Part model, mm, in its own coordinate system. A direction names the side the tool comes from. Round coordinates to 2 decimals unless told otherwise and drop trailing zeros. Write each loop counter-clockwise with the first axis right and the second up, starting at its lowest first coordinate (ties: lowest second). Pieces come first, ordered by that corner, then holes.
from build123d import *

# Parameters (mm, degrees)
F1_DEPTH = 5
F2_W     = 30
F2_H     = 15
F3_DEPTH = 3
F4_R     = 5.490381
F4_R_2   = 3
F5_DEPTH = 8


with BuildPart() as f1:
    # F0 (on Top) → F1 (new body)
    with BuildSketch(Plane.XY):
        Polygon((0, 25.980762), (-15, 0), (15, 0), align=None)
    extrude(amount=F1_DEPTH)

    # F2 (on face) → F3 (join)
    with BuildSketch(Plane.XZ):
        with Locations((0, 7.5)):
            Rectangle(F2_W, F2_H)
    extrude(amount=F3_DEPTH)

    # F4 (on face) → F5 (join)
    with BuildSketch(Plane.XY.offset(5)):
        with Locations((0, 15)):
            Circle(F4_R)
        with Locations((0, 15)):
            Circle(F4_R_2, mode=Mode.SUBTRACT)
    extrude(amount=F5_DEPTH)


solid = f1.part
Q1. Wall check: line 1 (Y direction, x = 0, z = 8.5); line 2 (Z direction, x = 4.75, y = 4.5); line 3 (Y direction, x = -13.75, z = 10.5). Give the ranges that are in metal, low to high.
Q2. Saw through at A-A, the plane z = 7. Write the cut outline in (x, y), and give its area (3 significant figures).
Q3. Saw through at C-C, the plane x = -2.5. Write the cut outline in (y, z), and give its area (3 significant figures).
Q4. Saw through at D-D, the plane x = 0.5. Write the cut outline in (y, z), and give its area (3 significant figures).
Q5. Saw through at B-B, the plane y = 11. Write the cut outline in (x, z).
Q6. Drop flat-ended pins along their axis: P1, Ø3.5, axis at x = 0, y = 15, coming from the +Z side; P2, Ø12, axis at x = -10.5, y = 18, coming from the +Z side; P3, Ø6, axis at y = 20.5, z = 7, coming from the +X side. Give the stop position or say it passes through.
Q7. Tool access for faces 4 (the flat face through (2.4, 12.6, 13)), 5 (the flat face through (0, 0, 10)), 6 (the flat face through (0, 15, 5)): list every direction of +Z, -Z, +X, -X, +Y, -Y with a clear straight run to the whole face (end or side of a thin tool).
Q8. Two-plate mould, pull along Y, no slides. Class faces 1 (the flat face through (0, 22, 5)), 2 (the flat face through (0, -3, 8)), 3 (the cylindrical face through (-1.19, 9.64, 8.94)): released by +Y, released by -Y, zero draft, split by the parting line, or undercut.
Computed:
1. line 1: y = -3 to 0, 9.51 to 12, 18 to 20.49
1. line 2: z = 0 to 5
1. line 3: y = -3 to 0
2. outline: (-15, -3) - (15, -3) - (15, 0) - (-15, 0) - close; circle Ø10.98 at (0, 15); hole circle Ø6 at (0, 15)
2. area: 156 mm2
3. outline: (-3, 0) - (21.65, 0) - (21.65, 5) - (19.89, 5) - (19.89, 13) - (16.66, 13) - (16.66, 5) - (13.34, 5) - (13.34, 13) - (10.11, 13) - (10.11, 5) - (0, 5) - (0, 15) - (-3, 15) - close
3. area: 205 mm2
4. outline: (-3, 0) - (25.11, 0) - (25.11, 5) - (20.47, 5) - (20.47, 13) - (17.96, 13) - (17.96, 5) - (12.04, 5) - (12.04, 13) - (9.53, 13) - (9.53, 5) - (0, 5) - (0, 15) - (-3, 15) - close
4. area: 211 mm2
5. outline: (-8.65, 0) - (8.65, 0) - (8.65, 5) - (3.76, 5) - (3.76, 13) - (-3.76, 13) - (-3.76, 5) - (-8.65, 5) - close
6. P1: stops at z = 5
6. P2: stops at z = 13
6. P3: stops at x = 4.89
7. face 4: +Z, +X, -X, +Y
7. face 5: +Z, +X, -X
7. face 6: +Z
8. face 1: zero draft
8. face 2: released by -Y
8. face 3: undercut
